Read the model definition and answer for the solid it produces. Units are mm, in the model's axes. A direction names the side the tool comes from. Give positions to 0.01 mm unless a question says otherwise; leave off trailing zeros. Write each loop counter-clockwise with the first axis right and the second up, starting at its lowest first coordinate (ties: lowest second). Pieces come first, ordered by that corner, then holes. Notation, with made-up numbers: M 0,62.25 L 20,62.25 A21 ccw 20,84.25 Z; hole C 13.25,-19 d7. An arc over 180 degrees is marked long. Use a Markdown table: item, result. Add a question column.
Item 1: A cutting plane is placed at A-A on z = 6. Determine the outline of the cut face in (x, y) (3 decimals).
Item 2: Given P1, Ø2, axis at y = -32.5, z = 3, coming from the +X side (3 decimals); P2, Ø14, axis at y = 15, z = 21, coming from the -X side (3 decimals); P3, Ø15, axis at x = 93.5, y = 9.5, coming from the -Z side, each flat-ended and moving along its own axis, determine where each tip first touches the part or whether it passes through.
Item 3: Consider probe 1 along X at (y, z) = (29, 1) (3 decimals); probe 2 along Z at (x, y) = (-17, -15.5) (3 decimals); probe 3 along Y at (x, z) = (68.5, 50). Determine where each line is inside the solid, lowest interval first. Write a range as [from, to].
Item 4: For faces 1 (the cylindrical face through (31.799, 16.547, 51.023)), 2 (the flat face through (60, -2, 61.925)), 3 (the flat face through (46, -25.4, 42)), 4 (the flat face through (46, 25.4, 42)), determine the directions among +Z, -Z, +X, -X, +Y, -Y from which every point of the face is accessible in a straight line to the end or side of a thin tool.
from build123d import *

# Parameters (mm, degrees)
F1_DEPTH = 63.5
F0_W     = 25.4
F0_H     = 19.05
F2_DEPTH = 25.4
F3_DEPTH = 7.9375
F5_R     = 6.35
F6_R     = 6.35
F7_R     = 6.35
F8_R     = 6.35


# Not quite as in the source:
# - a feature names something its author has since deleted; it is built from what else it names


with BuildPart() as f1:
    # F0 (on Front) → F1 (new body, symmetric)
    with BuildSketch(Plane.XZ):
        Polygon((22.225, 9.525), (-41.275, 9.525), (-41.275, -9.525), (41.275, -9.525), (41.275, 9.525), align=None)
    extrude(amount=F1_DEPTH, both=True)

    # F0 (on Front) → F2 (join, symmetric)
    with BuildSketch(Plane.XZ):
        with BuildLine():
            Line((22.225, 27.0002), (22.225, 9.525))
            Line((22.225, 9.525), (41.275, 9.525))
            Line((41.275, 9.525), (41.275, 27.0002))
            ThreePointArc((41.275, 27.0002), (45.9246798487, 38.2255201513), (57.15, 42.8752))
            Line((57.15, 42.8752), (60.325, 42.8752))
            Line((60.325, 42.8752), (60.325, 61.9252))
            Line((60.325, 61.9252), (57.15, 61.9252))
            add(Edge.make_bspline(
                [(54.5418748685, 61.8276792125), (55.4058435477, 61.8626883172), (56.2751659775, 61.8950651933), (57.15, 61.9252)],
                knots=[109.0113637744, 109.0113637744, 109.0113637744, 109.0113637744, 111.5045361635, 111.5045361635, 111.5045361635, 111.5045361635], degree=3))
            ThreePointArc((54.5418748685, 61.8276792125), (31.5487852318, 50.7559030498), (22.225, 27.0002))
        make_face()
        with Locations((73.025, 52.4002)):
            Rectangle(F0_W, F0_H)
    extrude(amount=F2_DEPTH, both=True)

    # F0 (on Front) → F3 (join, symmetric)
    with BuildSketch(Plane.XZ):
        with BuildLine():
            add(Edge.make_bspline(
                [(-41.275, 9.525), (-10.7751676539, 53.7339523615), (16.7657449889, 60.2969426058), (54.5418748685, 61.8276792125)],
                knots=[0, 0, 0, 0, 109.0113637744, 109.0113637744, 109.0113637744, 109.0113637744], degree=3))
            Line((-41.275, 9.525), (22.225, 9.525))
            Line((22.225, 9.525), (22.225, 27.0002))
            ThreePointArc((22.225, 27.0002), (31.5487852318, 50.7559030498), (54.5418748685, 61.8276792125))
        make_face()
    extrude(amount=F3_DEPTH, both=True)

    # F0 (on Front) → F4 (revolve)
    with BuildSketch(Plane.XZ):
        Polygon((85.725, 66.675), (85.725, 61.9252), (85.725, 42.8752), (85.725, 38.1), (111.125, 38.1), (111.125, 66.675), align=None)
    revolve(axis=Axis((85.725, 0, 52.3875), (0, 0, -1)))

    # F5
    f5_edges = [f1.edges().sort_by_distance(p)[0] for p in [
        (41.275, -63.5, 0),
    ]]
    fillet(f5_edges, radius=F5_R)

    # F6
    f6_edges = [f1.edges().sort_by_distance(p)[0] for p in [
        (-41.275, -63.5, 0),
    ]]
    fillet(f6_edges, radius=F6_R)

    # F7
    f7_edges = [f1.edges().sort_by_distance(p)[0] for p in [
        (-41.275, 63.5, 0),
    ]]
    fillet(f7_edges, radius=F7_R)

    # F8
    f8_edges = [f1.edges().sort_by_distance(p)[0] for p in [
        (41.275, 63.5, 0),
    ]]
    fillet(f8_edges, radius=F8_R)


solid = f1.part
Filled in:
| question | item | result |
|---|---|---|
| 1 | outline | M -41.275,-57.15 A6.35 ccw -34.925,-63.5 L 34.925,-63.5 A6.35 ccw 41.275,-57.15 L 41.275,57.15 A6.35 ccw 34.925,63.5 L -34.925,63.5 A6.35 ccw -41.275,57.15 Z |
| 2 | P1 | x = 41.275 |
| 2 | P2 | x = 22.225 |
| 2 | P3 | z = 38.1 |
| 3 | probe 1 | [-41.275, 41.275] |
| 3 | probe 2 | [-9.525, 9.525] |
| 3 | probe 3 | [-25.4, 25.4] |
| 4 | face 1 | +Z, -X, +Y |
| 4 | face 2 | +Z, -X |
| 4 | face 3 | +Z, +X, -X, -Y |
| 4 | face 4 | +Z, +X, -X, +Y |
